For this review, take the finished solid that the model builds, in its own axes (mm). A direction names the side the tool comes from. Round coordinates to 2 decimals unless told otherwise and drop trailing zeros. Write each loop counter-clockwise with the first axis right and the second up, starting at its lowest first coordinate (ties: lowest second). Pieces come first, ordered by that corner, then holes.
from build123d import *

# Parameters (mm, degrees)
F0_W        = 76.2
F0_H        = 152.4
F1_DEPTH    = 8.89
F2_T        = 8.636
F3_T1_DEPTH = 118.872
F3_T3_DEPTH = 195.072


# Not quite as in the source:
# - a fillet or chamfer that OpenCascade refuses, or shapes differently, is made with other operations: its cross-section is extruded or revolved along the edge and cut away or added


with BuildPart() as f1:
    # F0 (on Front) → F1 (new body)
    with BuildSketch(Plane.XZ):
        with Locations((1.7131138593, 3.2272135141)):
            Rectangle(F0_W, F0_H)
    extrude(amount=F1_DEPTH)

    # F2
    f2_openings = [f1.faces().sort_by_distance(p)[0] for p in [
        (1.713114, -8.89, 3.227214),
    ]]
    offset(amount=F2_T, openings=f2_openings, kind=Kind.INTERSECTION)

    # F3: fillet of radius 5.08 on 8 edges, made by hand

    # F3_s2 → F3_t1 (cut)
    with BuildSketch(Plane.YZ.offset(-57.7228861407)):
        with BuildLine():
            ThreePointArc((-8.89, -76.5287864859), (-7.4021024484, -80.1208889343), (-3.81, -81.6087864859))
            Line((-3.81, -81.6087864859), (-8.89, -81.6087864859))
            Line((-8.89, -81.6087864859), (-8.89, -76.5287864859))
        make_face()
        with BuildLine():
            ThreePointArc((-8.89, 82.9832135141), (-7.4021024484, 86.5753159626), (-3.81, 88.0632135141))
            Line((-3.81, 88.0632135141), (-8.89, 88.0632135141))
            Line((-8.89, 88.0632135141), (-8.89, 82.9832135141))
        make_face()
        with BuildLine():
            ThreePointArc((3.556, 88.0632135141), (7.1481024484, 86.5753159626), (8.636, 82.9832135141))
            Line((8.636, 82.9832135141), (8.636, 88.0632135141))
            Line((8.636, 88.0632135141), (3.556, 88.0632135141))
        make_face()
        with BuildLine():
            ThreePointArc((3.556, -81.6087864859), (7.1481024484, -80.1208889343), (8.636, -76.5287864859))
            Line((8.636, -76.5287864859), (8.636, -81.6087864859))
            Line((8.636, -81.6087864859), (3.556, -81.6087864859))
        make_face()
    extrude(amount=F3_T1_DEPTH, mode=Mode.SUBTRACT)

    # F3_s4 → F3_t3 (cut)
    with BuildSketch(Plane.XY.offset(-94.3087864859)):
        with BuildLine():
            ThreePointArc((43.3691138593, -8.89), (46.9612163077, -7.4021024484), (48.4491138593, -3.81))
            Line((48.4491138593, -3.81), (48.4491138593, -8.89))
            Line((48.4491138593, -8.89), (43.3691138593, -8.89))
        make_face()
        with BuildLine():
            ThreePointArc((-39.9428861407, -8.89), (-43.5349885891, -7.4021024484), (-45.0228861407, -3.81))
            Line((-45.0228861407, -3.81), (-45.0228861407, -8.89))
            Line((-45.0228861407, -8.89), (-39.9428861407, -8.89))
        make_face()
        with BuildLine():
            ThreePointArc((-45.0228861407, 3.556), (-43.5349885891, 7.1481024484), (-39.9428861407, 8.636))
            Line((-39.9428861407, 8.636), (-45.0228861407, 8.636))
            Line((-45.0228861407, 8.636), (-45.0228861407, 3.556))
        make_face()
        with BuildLine():
            ThreePointArc((48.4491138593, 3.556), (46.9612163077, 7.1481024484), (43.3691138593, 8.636))
            Line((43.3691138593, 8.636), (48.4491138593, 8.636))
            Line((48.4491138593, 8.636), (48.4491138593, 3.556))
        make_face()
    extrude(amount=F3_T3_DEPTH, mode=Mode.SUBTRACT)


solid = f1.part
(1) For line 1 along Z through (x, y) = (-6.5, -4); line 2 along X through (y, z) = (-3.5, 62); line 3 along Y through (x, z) = (-8.5, -31), list the stretches that pass through material, from the lowest coordinate up.
Geometry check:
line 1: z = -81.61 to -72.97, 79.43 to 88.06
line 2: x = -45.02 to -36.39, 39.81 to 48.45
line 3: y = 0 to 8.64
(2) We need section D-D, the plane y = 6.5. Give the boundary of the cut face in (x, z), and give its area (3 significant figures).
Geometry check:
outline: (-44.08, -80.67) - (47.51, -80.67) - (47.51, 87.12) - (-44.08, 87.12) - close
area: 15,400 mm2
(3) Mouldability with a two-part tool opening along X and no side actions: class faces 3 (the face through (1.059, 7.108, 86.615)), 4 (the face through (1, 0, 4)), 5 (the face through (-43.495, -7.441, 2.04)) as pulls with the +X half, pulls with the -X half, needs draft (parallel to the pull), parting line crosses it, or undercut.
Geometry check:
face 3: needs draft
face 4: undercut
face 5: pulls with the -X half
(4) For faces 1 (the face through (39.813, -4, 2)), 2 (the face through (1, 0, 88.063)), list the 3-axis set-ups (+Z, -Z, +X, -X, +Y, -Y) from which the entire face can be reached by the end or side of a thin tool; tool diameter is ignored.
Geometry check:
face 1: -Y
face 2: +Z, +X, -X, +Y, -Y
(5) For pin 1 Ø2.5 at (x, y) = (-3.5, -6) entering from +Z; pin 2 Ø4.5 at (y, z) = (-5.5, 7.5) entering from -X; pin 3 Ø2.5 at (x, y) = (-17.5, -6.5) entering from -Z; pin 4 Ø12 at (x, z) = (-19.5, 38) entering from -Y, all flat-tipped, find the tip position at first contact; note any pin that passes through.
Geometry check:
pin 1: stops at z = 87.98
pin 2: stops at x = -45.02
pin 3: stops at z = -81.4
pin 4: stops at y = 0
(6) We need section B-B, the plane z = 2. Give the boundary of the cut face in (x, y), and give its area (3 significant figures).
Geometry check:
outline: (-45.02, -3.81) arc R5.08 ccw to (-39.94, -8.89) - (-36.39, -8.89) - (-36.39, 0) - (39.81, 0) - (39.81, -8.89) - (43.37, -8.89) arc R5.08 ccw to (48.45, -3.81) - (48.45, 3.56) arc R5.08 ccw to (43.37, 8.64) - (-39.94, 8.64) arc R5.08 ccw to (-45.02, 3.56) - close
area: 939 mm2
(7) We need section C-C, the plane x = 4.5. Give the boundary of the cut face in (y, z), and give its area (3 significant figures).
Geometry check:
outline: (-8.89, -76.53) arc R5.08 ccw to (-3.81, -81.61) - (3.56, -81.61) arc R5.08 ccw to (8.64, -76.53) - (8.64, 82.98) arc R5.08 ccw to (3.56, 88.06) - (-3.81, 88.06) arc R5.08 ccw to (-8.89, 82.98) - (-8.89, 79.43) - (0, 79.43) - (0, -72.97) - (-8.89, -72.97) - close
area: 1,600 mm2
(8) We need section A-A, the plane y = -2.25. Give the boundary of the cut face in (x, z), and give its area (3 significant figures).
Geometry check:
outline: (-45.02, -81.61) - (48.45, -81.61) - (48.45, 88.06) - (-45.02, 88.06) - close; hole (-36.39, -72.97) - (39.81, -72.97) - (39.81, 79.43) - (-36.39, 79.43) - close
area: 4,250 mm2
